Autodesk Inventor part; units mm, degrees
ref_plane "YZ Plane" through (0, 0, 0) normal (1, 0, 0) x (0, 1, 0)
ref_plane "XZ Plane" through (0, 0, 0) normal (0, 1, 0) x (-1, 0, 0)
ref_plane "XY Plane" through (0, 0, 0) normal (0, 0, 1) x (1, 0, 0)
sketch "スケッチ1" plane through (0, 0, 0) normal (0, 0, 1) x (1, 0, 0)
  line L0 (56, 10) -> (-56, 10)
  line L1 (-56, 10) -> (-56, -10)
  line L2 (-56, -10) -> (56, -10)
  line L3 (56, -10) -> (56, 10)
  line L4 (56, 10) -> (-56, -10) construction
  line L5 (-56, 10) -> (56, -10) construction
  point P0 (0, 0)
  dimension "d0" = 112
  dimension "d1" = 20
extrude "押し出し1" add sketch "スケッチ1" along normal blind 1.5
sketch "スケッチ3" plane through (0, 0, 1.5) normal (0, 0, 1) x (1, 0, 0)
  line L0 (56, 10) -> (-56, 10)
  line L1 (-56, 10) -> (-56, -10)
  point P0 (0, 0)
  point P1 (-51, 5)
  point P2 (-51, -5)
  dimension "d10" = 10
  dimension "d11" = 5
  dimension "d12" = 5
hole "穴1" at (-51, 5, 1.5) at (-51, -5, 1.5) direction (0, 0, -1) diameter 3.1 end through all
sketch "スケッチ7" plane through (56, -10, 0) normal (1, 0, 0) x (0, 0, -1)
  line L0 (-1.5, 20) -> (0, 20)
  line L1 (0, 20) -> (0, 0)
  line L2 (0, 0) -> (-1.5, 0)
  line L3 (-1.5, 0) -> (-1.5, 20)
  point P0 (0, 10)
extrude "押し出し3" add sketch "スケッチ7" along normal blind 5
sketch "スケッチ8" plane through (0, 0, 1.5) normal (0, 0, 1) x (1, 0, 0)
  line L0 (55.2426, -4.2426) -> (51, 0)
  line L1 (55.2426, -4.2426) -> (61.2426, -4.2426) construction
  line L2 (61, 10) -> (61, -10)
  line L3 (-56, -10) -> (61, -10)
  point P0 (0, 0)
  point P1 (55.2426, 4.2424)
  point P2 (46.7576, 4.2424)
  point P3 (46.7576, -4.2426)
  dimension "d38" = 6
  dimension "d39" = 135
  dimension "d40" = 10
  dimension "d41" = 10
  dimension "d52" = 8.485
  dimension "d53" = 8.485
hole "穴4" at (55.2426, -4.2426, 1.5) at (46.7576, -4.2426, 1.5) at (46.7576, 4.2424, 1.5) at (55.2426, 4.2424, 1.5) direction (0, 0, -1) diameter 2.1 end through all
properties part number "Fork 4 right ver2.1" material "アルミニウム 5052 H32"
Source: CAD feature listing. Evaluate the final solid. Frame: model axes, mm. Give positions to 0.01 mm unless a question says otherwise; leave off trailing zeros. Loops run counter-clockwise (first coordinate to the right, second up) from the corner with the lowest first, then second, coordinate; pieces in that order, holes last. Notation, with made-up numbers: (7, -24) -> (31, -24) arc R14 cw to (31, -3) -> close; hole circle Ø3 at (-10.75, 25.25). An arc over 180 degrees is marked (long way). Put each result on its own line as item: value. Start each with the question number.
1) Material intervals for probe 1 along Y at (x, z) = (-51, 0.9); probe 2 along X at (y, z) = (-4, 0.4); probe 3 along X at (y, z) = (4.5, 1.25), sorted ascending.
2) Cut plane A-A (x = -51). Return loops of the section in (y, z), then the cut area to 3 significant figures.
3) Contact query for flat-ended pins moving along their axis: P1, Ø8, axis at x = 21, y = 4, coming from the -Z side; P2, Ø1.3, axis at x = 55.24, y = 4.24, coming from the -Z side. Output: stop coordinate, or through.
Results are:
1. probe 1: y = -10 to -6.55, -3.45 to 3.45, 6.55 to 10
1. probe 2: x = -56 to -52.18, -49.82 to 45.74, 47.78 to 54.22, 56.26 to 61
1. probe 3: x = -56 to -52.47, -49.53 to 45.74, 47.78 to 54.22, 56.26 to 61
2. outline: (-10, 0) -> (-6.55, 0) -> (-6.55, 1.5) -> (-10, 1.5) -> close; (-3.45, 0) -> (3.45, 0) -> (3.45, 1.5) -> (-3.45, 1.5) -> close; (6.55, 0) -> (10, 0) -> (10, 1.5) -> (6.55, 1.5) -> close
2. area: 20.7 mm2
3. P1: stops at z = 0
3. P2: passes through
